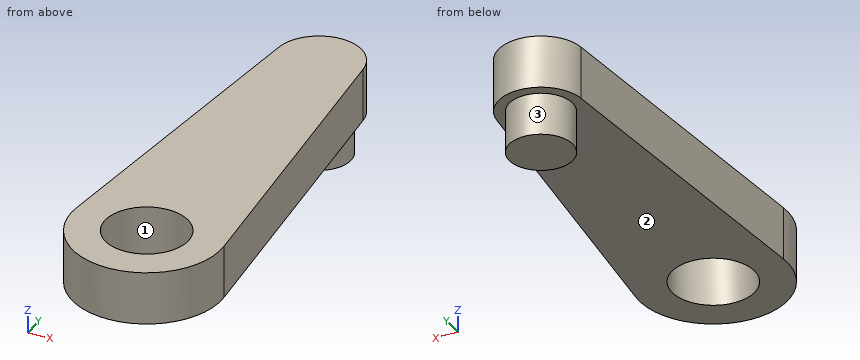
Autodesk Inventor part; units mm, degrees
ref_plane "YZ Plane" through (0, 0, 0) normal (1, 0, 0) x (0, 1, 0)
ref_plane "XZ Plane" through (0, 0, 0) normal (0, 1, 0) x (-1, 0, 0)
ref_plane "XY Plane" through (0, 0, 0) normal (0, 0, 1) x (1, 0, 0)
sketch "Эскиз1" plane through (0, 0, 0) normal (0, 0, 1) x (1, 0, 0)
  circle A0 centre (0, 0) radius 4
  arc A1 (-13.2, 4.5) -> (-13.2, -4.5) centre (-13.2, 0) ccw
  line L0 (-13.2, -4.5) -> (1.3, -4.5)
  arc A2 (1.3, -4.5) -> (1.3, 4.5) centre (1.3, 0) ccw
  line L1 (1.3, 4.5) -> (-13.2, 4.5)
  circle A3 centre (0, 6.5601) radius 1.1
  arc A4 (-8.1687, 23.1585) -> (8.1687, 23.1585) centre (0, 35.5) ccw
  arc A5 (10.1004, 20.2399) -> (8.1687, 23.1585) centre (9.1346, 21.6992) ccw
  arc A6 (-10.1004, 20.2399) -> (10.1004, 20.2399) centre (0, 35.5) ccw
  arc A7 (-8.1687, 23.1585) -> (-10.1004, 20.2399) centre (-9.1346, 21.6992) ccw
  line L2 (13.75, 27.1) -> (13.75, 10.8)
  line L3 (13.75, 27.1) -> (-13.75, 27.1)
  line L4 (-13.75, 27.1) -> (-13.75, 10.8)
  line L5 (-13.75, 10.8) -> (-0.7414, 4.9199)
  arc A8 (-0.7414, 4.9199) -> (0.7414, 4.9199) centre (0, 6.5601) ccw
  line L6 (0.7414, 4.9199) -> (13.75, 10.8)
  circle A9 centre (0, 0) radius 14.9209
  circle A10 centre (-9.898, 8.3054) radius 2
  circle A11 centre (0, 0) radius 1.5
  circle A12 centre (0, 0) radius 3.5
  line L7 (-86.0992, 75.6487) -> (86.0992, -4.6487)
  line L8 (-1.991, 16.0319) -> (-3.4843, 0.3314)
  line L9 (3.4843, 0.3314) -> (1.991, 16.0319)
  circle A13 centre (0, 6.5601) radius 1.25
  line L10 (1.25, 15.8425) -> (1.25, 6.5601)
  line L11 (-1.25, 6.5601) -> (-1.25, 15.8425)
  arc A14 (14.6884, 10.9864) -> (-14.6884, 10.9864) centre (0, 0) ccw
  arc A15 (14.8244, 8.1933) -> (14.6884, 10.9864) centre (12.6864, 9.489) ccw
  arc A16 (-14.6884, 10.9864) -> (-15.006, 8.5565) centre (-12.6864, 9.489) ccw
  circle A17 centre (0, 0) radius 15.8425
  circle A18 centre (0, 15.8425) radius 1.25
  circle A19 centre (0, 15.8425) radius 2
  line L12 (0, 7.2054) -> (0, 9.4054)
  line L13 (0, -12.9209) -> (0, 12.9209)
  point P0 (0, 0)
  point P1 (86.0992, -4.6487)
  point P2 (-1.25, 15.7932)
  point P3 (-1.249, 15.7932)
  point P4 (1.249, 15.7932)
  point P5 (1.25, 15.7932)
  point P6 (2.0213, 15.7131)
  point P7 (1.996, 15.7163)
  point P8 (-1.996, 15.7163)
  point P9 (-2.0213, 15.7131)
  dimension "d0" = 4
  dimension "d1" = 3
  dimension "d2" = 7
  dimension "d6" = 2.5
  dimension "d7" = 2.5
  dimension "d8" = 4
extrude "Выдавливание1" add sketch "Эскиз1" along normal blind 2.5 contours L9 A12 L13 A0 | A0 L13 L1 A2 L9 | L13 A12 L8 A0 | A0 L8 L1 L13 | A12 L13 A11 | A2 L1 L13 A8 L6 L9 | A12 L13 A11 | L1 L8 L5 A8 L13 | L6 A8 L13 A13 L10 A19 A9 L9 | A8 L5 L8 A9 A19 L11 A13 L13 | A9 A19 A17 L9 | L13 A3 L12 A13 | A13 L12 A3 L13 | A19 L10 A9 | A9 L10 A17 A19 | A17 A19 L9 | L8 A17 A19 A9 | L11 A19 L10 A13 | L13 L12 A3 | A3 L12 L13 | L10 A19 L11 A9 A18 | A9 A18 L10 | A17 L10 A18 L11 A19 A6 | A19 A17 L11 A9 | A9 L11 A19 | L8 A19 A17 | A18 A9 | A9 A18 A17 | A17 L11 A18 L10 | A6 A19 | L11 A18 A9 picked at (0.3204, 3.7943) picked at (-0.3204, 3.7943)
sketch "Эскиз2" plane through (0, 0, 0) normal (0, 0, -1) x (-1, 0, 0)
  circle A0 centre (0, 0) radius 14.9209
  arc A1 (1.991, 16.0319) -> (-1.991, 16.0319) centre (0, 12.9209) ccw
  circle A2 centre (0, 0) radius 1.95
  arc A3 (-3.4843, 0.3314) -> (3.4843, 0.3314) centre (0, 0) ccw
  line L0 (1.991, 16.0319) -> (3.4843, 0.3314)
  arc A4 (1.991, 16.0319) -> (-1.991, 16.0319) centre (0, 15.8425) ccw
  line L1 (-3.4843, 0.3314) -> (-1.991, 16.0319)
  point P0 (0, 0)
  dimension "d9" = 3.9
extrude "Выдавливание2" cut sketch "Эскиз2" against normal blind 3 contours A2
sketch "Эскиз3" plane through (0, 0, 0) normal (0, 0, -1) x (-1, 0, 0)
  circle A0 centre (0, 0) radius 1.95
  arc A1 (-3.4843, 0.3314) -> (3.4843, 0.3314) centre (0, 0) ccw
  line L0 (1.991, 16.0319) -> (3.4843, 0.3314)
  arc A2 (1.991, 16.0319) -> (-1.991, 16.0319) centre (0, 15.8425) ccw
  line L1 (-3.4843, 0.3314) -> (-1.991, 16.0319)
  circle A3 centre (0, 15.8425) radius 1.5
  point P0 (0, 0)
  dimension "d12" = 3
extrude "Выдавливание3" add sketch "Эскиз3" along normal blind 2 contours A3
properties part number "shatun_lidar"
Here's how the part is built. I have some questions about the finished solid (model axes, mm). Face numbers are marked on the shaded views. Round coordinates to 2 decimals unless told otherwise and drop trailing zeros. Order: outer loops, then holes, each group sorted by start corner. A loop starts at its lowest first (then second) coordinate and runs counter-clockwise, first axis right, second up. Notation, with made-up numbers: (43, 65.5) -> (76, 65.5) arc R20 cw to (76, 80.5) -> close; hole circle Ø6 at (4.5, 86.25). An arc over 180 degrees is marked (long way). Return JSON: item names as keys, results as strings.
Q1. If we section it at B-B on x = 0: List the corners of the cut face in (y, z) for me.
Filled sheet:
{"outline": "(-3.5, 0) -> (-1.95, 0) -> (-1.95, 2.5) -> (-3.5, 2.5) -> close; (1.95, 0) -> (14.34, 0) -> (14.34, -2) -> (17.34, -2) -> (17.34, 0) -> (17.84, 0) -> (17.84, 2.5) -> (1.95, 2.5) -> close"}
Q2. If we section it at C-C on z = 0.7: List the corners of the cut face in (x, y) for me, plus the area to 3 significant figures.
Filled sheet:
{"outline": "(-3.48, 0.33) arc R3.5 ccw (long way) to (3.48, 0.33) -> (1.99, 16.03) arc R2 ccw to (-1.99, 16.03) -> close; hole circle Ø3.9 at (0, 0)", "area": "101 mm^2"}
Q3. I need wall thicknesses on line 1 along Y through (x, z) = (0, 0.5); line 2 along Z through (x, y) = (-1.75, 6.5); line 3 along Y through (x, z) = (-1.5, 0.75). Which ranges of each line are inside material? Lowest first, please. Write a range as from..to.
Filled sheet:
{"line 1": "y = -3.5..-1.95, 1.95..17.84", "line 2": "z = 0..2.5", "line 3": "y = -3.16..-1.25, 1.25..17.17"}
Q4. If we mould it in two halves opening along X, with no side actions, what happens to the marked faces 1, 2 and 3? For each: released by +X, released by -X, zero draft, split by the parting line, or undercut.
Filled sheet:
{"face 1": "undercut", "face 2": "zero draft", "face 3": "split by the parting line"}
Q5. For pin 1 Ø4 at (x, y) = (2.5, 3) entering from -Z, with a flat end and sliding along its axis, tell me the tip position at first contact or that it passes through.
Filled sheet:
{"pin 1": "stops at z = 0"}
Q6. If we section it at D-D on y = 12.75: List the corners of the cut face in (x, z) for me.
Filled sheet:
{"outline": "(-2.3, 0) -> (2.3, 0) -> (2.3, 2.5) -> (-2.3, 2.5) -> close"}
Q7. If we section it at A-A on y = 0: List the corners of the cut face in (x, z) for me.
Filled sheet:
{"outline": "(-3.5, 0) -> (-1.95, 0) -> (-1.95, 2.5) -> (-3.5, 2.5) -> close; (1.95, 0) -> (3.5, 0) -> (3.5, 2.5) -> (1.95, 2.5) -> close"}
